from build123d import *

# Parameters (mm, degrees)
BOSS_EXTRUDE1_DEPTH     = 12
CUT_EXTRUDE1_DEPTH      = 50.623583103
CUT_EXTRUDE1_DEPTH_BACK = 50.623583103
SKETCH2_R               = 1.25


with BuildPart() as part:
    # Sketch1 → Boss-Extrude1 (new body)
    with BuildSketch(Plane.XY):
        with BuildLine():
            Line((-12.5, 0), (12.5, 0))
            Line((12.5, 0), (12.5, 46.5))
            Line((12.5, 46.5), (4.5, 46.5))
            ThreePointArc((4.5, 46.5), (0, 42), (-4.5, 46.5))
            Line((-4.5, 46.5), (-12.5, 46.5))
            Line((-12.5, 46.5), (-12.5, 0))
        make_face()
    extrude(amount=BOSS_EXTRUDE1_DEPTH)

    # Sketch2 → Cut-Extrude1 (cut, two sides: drawn at the far end of the back side and taken through both)
    with BuildSketch(Plane(origin=(0, 0, 0), x_dir=(-1, 0, 0), z_dir=(0, 0, -1)).offset(-CUT_EXTRUDE1_DEPTH_BACK)):
        with Locations((-7.4, 25)):
            Circle(SKETCH2_R)
        with Locations((2.1, 25)):
            Circle(SKETCH2_R)
    extrude(amount=CUT_EXTRUDE1_DEPTH + CUT_EXTRUDE1_DEPTH_BACK, mode=Mode.SUBTRACT)


solid = part.part
Build history of the part. All positions in model axes, mm. Give positions to 0.01 mm unless a question says otherwise; leave off trailing zeros. Order: outer loops, then holes, each group sorted by start corner. A loop starts at its lowest first (then second) coordinate and runs counter-clockwise, first axis right, second up. Notation, with made-up numbers: M 54.5,29 L 95.5,29 A10 cw 95.5,33 Z; hole C 35.5,60.25 d4. An arc over 180 degrees is marked long. Put each result on its own line as item: value.
Item 1: Slice it at B-B, the plane x = 7.4. Write the cut outline in (y, z).
From the geometry:
outline: M 0,0 L 23.75,0 L 23.75,12 L 0,12 Z; M 26.25,0 L 46.5,0 L 46.5,12 L 26.25,12 Z
Item 2: Slice it at C-C, the plane z = 2. Write the cut outline in (x, y), plus the area to 3 significant figures.
From the geometry:
outline: M -12.5,0 L 12.5,0 L 12.5,46.5 L 4.5,46.5 A4.5 cw -4.5,46.5 L -12.5,46.5 Z; hole C -2.1,25 d2.5; hole C 7.4,25 d2.5
area: 1,120 mm2
Item 3: Slice it at A-A, the plane y = 25. Write the cut outline in (x, z), plus the area to 3 significant figures.
From the geometry:
outline: M -12.5,0 L -3.35,0 L -3.35,12 L -12.5,12 Z; M -0.85,0 L 6.15,0 L 6.15,12 L -0.85,12 Z; M 8.65,0 L 12.5,0 L 12.5,12 L 8.65,12 Z
area: 240 mm2
Item 4: Probe line 1 (X direction, y = 25, z = 2.5); line 2 (Y direction, x = 8.5, z = 6.25); line 3 (Y direction, x = -3, z = 4.25). List the from-to ranges inside material, lowest first. Write a range as [from, to].
From the geometry:
line 1: x = [-12.5, -3.35], [-0.85, 6.15], [8.65, 12.5]
line 2: y = [0, 24.41], [25.59, 46.5]
line 3: y = [0, 24.13], [25.87, 43.15]
Item 5: Slice it at D-D, the plane x = -1.5. Write the cut outline in (y, z).
From the geometry:
outline: M 0,0 L 23.9,0 L 23.9,12 L 0,12 Z; M 26.1,0 L 42.26,0 L 42.26,12 L 26.1,12 Z
Item 6: Two-plate mould, pull along X, no slides. Class faces 1 (the flat face through (12.5, 23, 6)), 2 (the flat face through (9, 46.5, 6)), 3 (the cylindrical face through (-1.83, 23.78, 6.08)), 4 (the cylindrical face through (0, 42, 6)): +X half, -X half, draft (parallel to the pull), parting line (faces both ways), or undercut.
From the geometry:
face 1: +X half
face 2: draft
face 3: undercut
face 4: undercut
